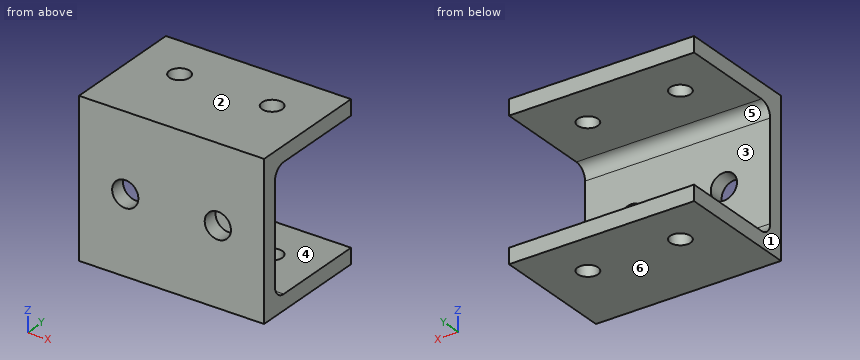
from build123d import *

# Parameters (mm, degrees)
EXTRUDE_1_DEPTH     = 60
SKETCH_2_R          = 4.25
CUT_EXTRUDE_1_DEPTH = 88.749643874
SKETCH_3_R          = 3.3
CUT_EXTRUDE_2_DEPTH = 88.749643874
FILLET_1_R          = 4


with BuildPart() as part:
    # 草圖1 → 填料-伸長1 (new body)
    with BuildSketch(Plane(origin=(0, 0, 0), x_dir=(0, 0, -1), z_dir=(1, 0, 0))):
        Polygon((0, 0), (50, 0), (50, 40), (45, 40), (45, 5), (5, 5), (5, 40), (0, 40), align=None)
    extrude(amount=EXTRUDE_1_DEPTH)

    # 草圖2 → 除料-伸長1 (cut, through all)
    with BuildSketch(Plane(origin=(0, 0, 0), x_dir=(1, 0, 0), z_dir=(0, 1, 0))):
        with Locations(Location((15, 25, 0), (0, 0, 90))):
            Circle(SKETCH_2_R)
        with Locations(Location((45, 25, 0), (0, 0, 90))):
            Circle(SKETCH_2_R)
    extrude(amount=CUT_EXTRUDE_1_DEPTH, mode=Mode.SUBTRACT)

    # 草圖3 → 除料-伸長2 (cut, through all)
    with BuildSketch(Plane.XY):
        with Locations((15, 25)):
            Circle(SKETCH_3_R)
        with Locations((45, 25)):
            Circle(SKETCH_3_R)
    extrude(amount=-CUT_EXTRUDE_2_DEPTH, mode=Mode.SUBTRACT)

    # 圓角1
    fillet_1_edges = [part.edges().sort_by_distance(p)[0] for p in [
        (30, 5, -5),
        (30, 5, -45),
    ]]
    fillet(fillet_1_edges, radius=FILLET_1_R)


solid = part.part
Verification items for the finished model (mm, model axes). Face numbers are marked on the shaded views. A direction names the side the tool comes from. Coordinates: 2 decimals unless noted, no trailing zeros. Order: outer loops, then holes, each group sorted by start corner. A loop starts at its lowest first (then second) coordinate and runs counter-clockwise, first axis right, second up.
1. Go/stop test with a flat-tipped pin: pin 1 Ø9.5 at (x, z) = (30.5, -22.5) entering from +Y. Record where the tip stops, or that it passes through.
Results found:
pin 1: stops at y = 5
2. Set-up check for the marked faces 5 and 6: record each of +Z, -Z, +X, -X, +Y, -Y from which the full face is reachable in a straight line by a thin tool's end or side.
Results found:
face 5: +X, -X, +Y
face 6: -Z, +X, -X, +Y, -Y
3. Sectioned sample at B-B, the plane x = 45. Record the cut outline in (y, z).
Results found:
outline: (0, -50) - (21.7, -50) - (21.7, -45) - (9, -45) arc R4 cw to (5, -41) - (5, -29.25) - (0, -29.25) - close; (0, -20.75) - (5, -20.75) - (5, -9) arc R4 cw to (9, -5) - (21.7, -5) - (21.7, 0) - (0, 0) - close; (28.3, -50) - (40, -50) - (40, -45) - (28.3, -45) - close; (28.3, -5) - (40, -5) - (40, 0) - (28.3, 0) - close
4. Scan lines: line 1 (X direction, y = 1.7, z = -25); line 2 (Z direction, x = 54, y = 20); line 3 (Y direction, x = 45, z = -1). Record each from-to range of solid material in increasing order.
Results found:
line 1: x = 0 to 10.75, 19.25 to 40.75, 49.25 to 60
line 2: z = -50 to -45, -5 to 0
line 3: y = 0 to 21.7, 28.3 to 40
5. Sectioned sample at D-D, the plane y = 25. Record the cut outline in (x, z), and give its area (3 significant figures).
Results found:
outline: (0, -50) - (11.7, -50) - (11.7, -45) - (0, -45) - close; (0, -5) - (11.7, -5) - (11.7, 0) - (0, 0) - close; (18.3, -50) - (41.7, -50) - (41.7, -45) - (18.3, -45) - close; (18.3, -5) - (41.7, -5) - (41.7, 0) - (18.3, 0) - close; (48.3, -50) - (60, -50) - (60, -45) - (48.3, -45) - close; (48.3, -5) - (60, -5) - (60, 0) - (48.3, 0) - close
area: 468 mm2
6. Sectioned sample at A-A, the plane z = -25. Record the cut outline in (x, y).
Results found:
outline: (0, 0) - (10.75, 0) - (10.75, 5) - (0, 5) - close; (19.25, 0) - (40.75, 0) - (40.75, 5) - (19.25, 5) - close; (49.25, 0) - (60, 0) - (60, 5) - (49.25, 5) - close
7. Release check for a two-part mould opening along Z. For the marked faces 1, 2, 3 and 4 record: +Z half, -Z half, draft (parallel to the pull), parting line (faces both ways), or undercut.
Results found:
face 1: draft
face 2: +Z half
face 3: undercut
face 4: undercut
8. Sectioned sample at C-C, the plane y = 15.5. Record the cut outline in (x, z).
Results found:
outline: (0, -50) - (60, -50) - (60, -45) - (0, -45) - close; (0, -5) - (60, -5) - (60, 0) - (0, 0) - close
